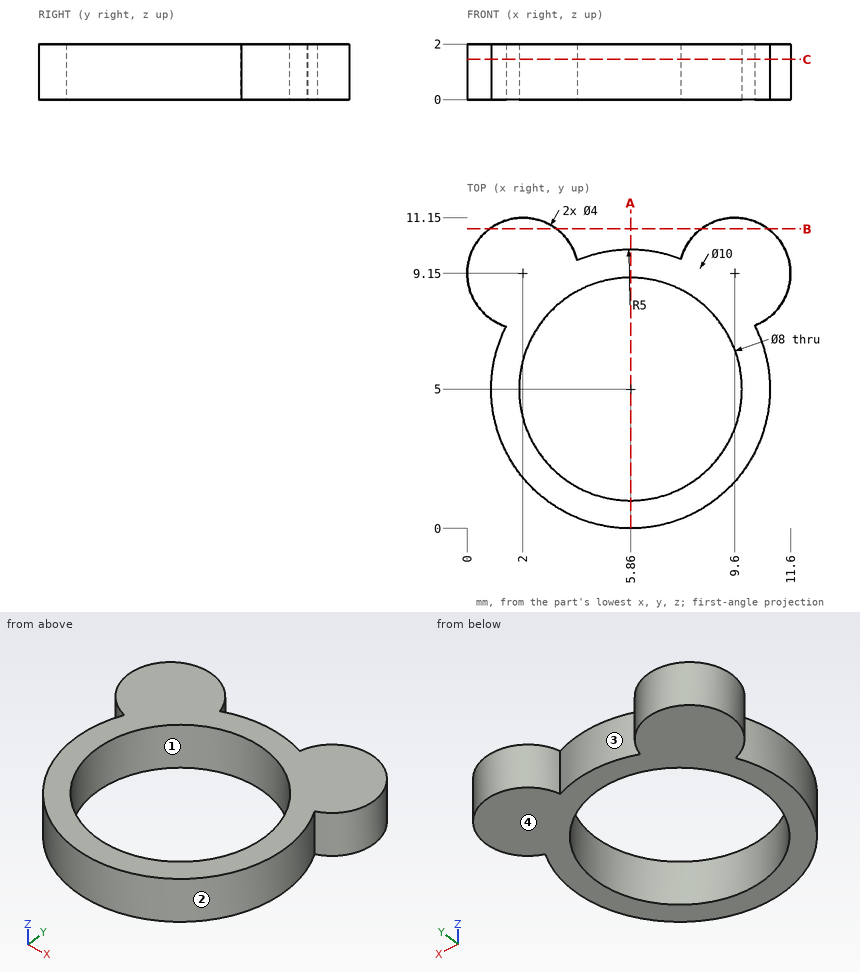
Study the drawing (mm; zero at the part's minimum x, y, z) and answer. Coordinates: 2 decimals unless noted, no trailing zeros. Loops run counter-clockwise (first coordinate to the right, second up) from the corner with the lowest first, then second, coordinate; pieces in that order, holes last. Notation, with made-up numbers: M 85.5,8 L 129.5,8 A24 cw 129.5,32 Z; hole C -3.75,36.5 d9. An arc over 180 degrees is marked long. Answer in a Markdown table with one row per item. Add a question column.
1. Find section C-C, the plane z = 1.45. Write down the section's boundary in (x, y).
2. The mould has two halves that part along X. Classify the marked faces 1, 2, 3 and 4: pulls with the +X half, pulls with the -X half, needs draft (parallel to the pull), parting line crosses it, or undercut.
3. Find section A-A, the plane x = 5.86. Write down the section's boundary in (y, z).
4. Find section B-B, the plane y = 10.75. Write down the section's boundary in (x, z).
5. Consider L1, parallel to Y at x = 5.86, z = 0.65; L2, parallel to X at y = 8.5, z = 0.9; L3, parallel to Y at x = 4.5, z = 0.55. Determine where each line is inside the solid, lowest interval first.
Reported:
| question | item | result |
|---|---|---|
| 1 | outline | M 1.39,7.24 A5 ccw long 10.31,7.28 A2 ccw long 7.67,9.66 A5 ccw 3.94,9.62 A2 ccw long Z; hole C 5.86,5 d8 |
| 2 | face 1 | undercut |
| 2 | face 2 | parting line crosses it |
| 2 | face 3 | undercut |
| 2 | face 4 | needs draft |
| 3 | outline | M 0,0 L 1,0 L 1,2 L 0,2 Z; M 9,0 L 10,0 L 10,2 L 9,2 Z |
| 4 | outline | M 0.8,0 L 3.2,0 L 3.2,2 L 0.8,2 Z; M 8.4,0 L 10.8,0 L 10.8,2 L 8.4,2 Z |
| 5 | L1 | y = 0 to 1, 9 to 10 |
| 5 | L2 | x = 0.11 to 3.92, 7.8 to 11.49 |
| 5 | L3 | y = 0.19 to 1.24, 8.76 to 9.81 |
